Can you work these out from the model? Positions are in its coordinate system, mm. Face numbers are marked on the shaded views. A direction names the side the tool comes from. Give positions to 0.01 mm unless a question says otherwise; leave off trailing zeros. Loops run counter-clockwise (first coordinate to the right, second up) from the corner with the lowest first, then second, coordinate; pieces in that order, holes last. Notation, with made-up numbers: M 43,9.5 L 55,9.5 A13 ccw 55,15.5 Z; hole C -7,26.5 d9. An arc over 180 degrees is marked long. Put each result on its own line as item: value. Start each with the question number.
1) For the marked faces 1 and 2, which set-ups out of +Z, -Z, +X, -X, +Y, -Y let a thin tool reach every point of the face, with its end or its side?
2) Imagine slicing it at D-D (z = 7.5). Write out the boundary of the cut face in (x, y), then the cut area to 3 significant figures.
3) Imagine slicing it at A-A (z = 1.25). Write out the boundary of the cut face in (x, y), then the cut area to 3 significant figures.
4) Imagine slicing it at B-B (x = -1.27). Write out the boundary of the cut face in (y, z), then the cut area to 3 significant figures.
5) Please list where these lines run through material, in increasing order: line 1 along Y through (x, z) = (3.81, 1.5); line 2 along Z through (x, y) = (5.25, 0.4); line 3 along Y through (x, z) = (3.5, 5.5). Write a range as from..to.
6) For P1, Ø1, axis at x = -2.5, y = -1, coming from the +Z side; P2, Ø1, axis at y = 1.5, z = 2, coming from the -X side, each with a flat end and sliding along its axis, tell me the tip position at first contact or that it passes through.
7) Imagine slicing it at C-C (x = -4.5). Write out the boundary of the cut face in (y, z).
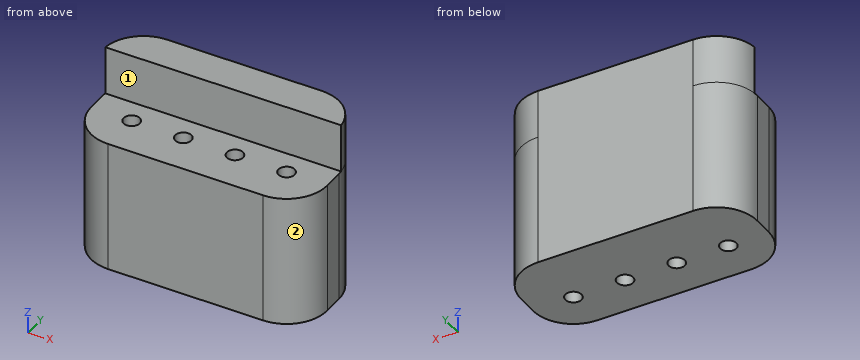
from build123d import *

# Parameters (mm, degrees)
SKETCH_R     = 0.4
PAD_DEPTH    = 6.5
PAD001_DEPTH = 2.4


with BuildPart() as part:
    # Sketch → Pad (new body)
    with BuildSketch(Plane.XY):
        with BuildLine():
            Line((-3.81, -2), (3.81, -2))
            ThreePointArc((3.81, -2), (5.224214, -1.414214), (5.81, 0))
            Line((5.81, 0), (5.81, 1))
            ThreePointArc((5.81, 1), (5.224214, 2.414214), (3.81, 3))
            Line((3.81, 3), (-3.81, 3))
            ThreePointArc((-3.81, 3), (-5.224214, 2.414214), (-5.81, 1))
            Line((-5.81, 0), (-5.81, 1))
            ThreePointArc((-5.81, 0), (-5.224214, -1.414214), (-3.81, -2))
        make_face()
        with Locations((-3.81, 0)):
            Circle(SKETCH_R, mode=Mode.SUBTRACT)
        with Locations((-1.27, 0)):
            Circle(SKETCH_R, mode=Mode.SUBTRACT)
        with Locations((1.27, 0)):
            Circle(SKETCH_R, mode=Mode.SUBTRACT)
        with Locations((3.81, 0)):
            Circle(SKETCH_R, mode=Mode.SUBTRACT)
    extrude(amount=PAD_DEPTH)

    # Sketch001 → Pad001 (join)
    with BuildSketch(Plane.XY.offset(6.5)):
        with BuildLine():
            ThreePointArc((-3.81, 3), (-5.151641, 2.48324), (-5.799975, 1.2))
            Line((-5.799975, 1.2), (5.799975, 1.2))
            ThreePointArc((5.799975, 1.2), (5.151641, 2.48324), (3.81, 3))
            Line((-3.81, 3), (3.81, 3))
        make_face()
    extrude(amount=PAD001_DEPTH)


solid = part.part
Recorded:
1. face 1: +Z, +X, -X, -Y
1. face 2: +Z, -Z, +X, -Y
2. outline: M -5.8,1.2 L 5.8,1.2 A2 ccw 3.81,3 L -3.81,3 A2 ccw Z
2. area: 19.2 mm²
3. outline: M -5.81,0 A2 ccw -3.81,-2 L 3.81,-2 A2 ccw 5.81,0 L 5.81,1 A2 ccw 3.81,3 L -3.81,3 A2 ccw -5.81,1 Z; hole C -3.81,0 d0.8; hole C -1.27,0 d0.8; hole C 1.27,0 d0.8; hole C 3.81,0 d0.8
3. area: 52.7 mm²
4. outline: M -2,0 L -0.4,0 L -0.4,6.5 L -2,6.5 Z; M 0.4,0 L 3,0 L 3,8.9 L 1.2,8.9 L 1.2,6.5 L 0.4,6.5 Z
4. area: 31.6 mm²
5. line 1: -2..-0.4, 0.4..3
5. line 2: 0..6.5
5. line 3: -2..-0.25, 0.25..3
6. P1: z = 6.5
6. P2: x = -5.81
7. outline: M -1.88,0 L 2.88,0 L 2.88,8.9 L 1.2,8.9 L 1.2,6.5 L -1.88,6.5 Z
